```python
from build123d import *

# Parameters (mm, degrees)
F5_DEPTH = 25
F6_DEPTH = 25
F7_COUNT = 7


with BuildPart() as f5:
    # F3 (on Front) → F5 (new body)
    with BuildSketch(Plane.XZ):
        with BuildLine():
            ThreePointArc((-5, 29.5803989155), (-19.364916731, -22.9128784748), (30, 0))
            ThreePointArc((30, 0), (22.9128784748, 19.364916731), (5, 29.5803989155))
            ThreePointArc((5, 29.5803989155), (0, 30), (-5, 29.5803989155))
        make_face()
    extrude(amount=F5_DEPTH)



with BuildPart() as f6:
    # F3 (on Front) → F6 (new body)
    with BuildSketch(Plane.XZ):
        with BuildLine():
            ThreePointArc((-5, 29.5803989155), (0, 30), (5, 29.5803989155))
            Line((5, 29.5803989155), (1.0056277868, 30.2555710497))
            Line((1.0056277868, 30.2555710497), (0, 30.2555710497))
            Line((0, 30.2555710497), (-1.0056277868, 30.2555710497))
            Line((-1.0056277868, 30.2555710497), (-5, 29.5803989155))
        make_face()
    extrude(amount=F6_DEPTH)


with BuildPart() as f5_1:
    add(f5.part)

    add(f6.part)  # F7 merges F6
    # F7: F6, F5 ×7 about axis
    f7_axis = Axis((0, 33.5468817502, 0), (0, 1, 0))
    for i in range(1, F7_COUNT):
        add(f6.part.rotate(f7_axis, i * 360 / F7_COUNT))
        add(f5.part.rotate(f7_axis, i * 360 / F7_COUNT))


solid = f5_1.part
```
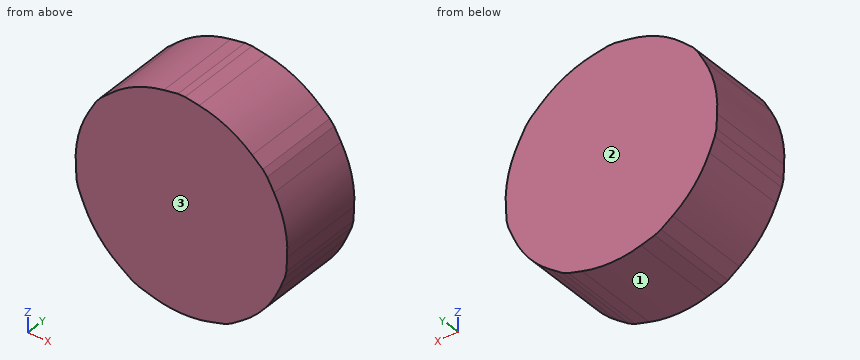
Design review of the part built by this model. Coordinates are the model's own, in mm. Face numbers are marked on the shaded views. Round coordinates to 2 decimals unless told otherwise and drop trailing zeros. Write each loop counter-clockwise with the first axis right and the second up, starting at its lowest first coordinate (ties: lowest second). Pieces come first, ordered by that corner, then holes.
Item 1: We need section B-B on x = 21. Write out the cut boundary in (y, z).
Item 2: Clearance check with flat-ended pins moving along their axes: pin 1 Ø10 at (y, z) = (-21, -15) entering from -X; pin 2 Ø6 at (x, y) = (21, -3) entering from +Z; pin 3 Ø10 at (y, z) = (-16, -10) entering from +X. State where each tip first meets the part, or that it passes through.
Item 3: For probe 1 along X at (y, z) = (-6.75, 14.5); probe 2 along X at (y, z) = (-14.5, 1.5); probe 3 along Z at (x, y) = (-3, -12.75), list the stretches that pass through material, from the lowest coordinate up.
Item 4: The part is to be moulded in two halves that separate along Y. For the marked faces 1, 2 and 3, say which applies: +Y half, -Y half, draft (parallel to the pull), parting line (faces both ways), or undercut.
Item 5: We need section C-C on z = -22. Write out the cut boundary in (x, y).
Item 6: We need section A-A on y = -22. Write out the cut boundary in (x, z).
Returned:
1. outline: (-25, -21.42) - (0, -21.42) - (0, 21.47) - (-25, 21.47) - close
2. pin 1: stops at x = -28.33
2. pin 2: stops at z = 24
2. pin 3: stops at x = 29.76
3. probe 1: x = -26.26 to 26.26
3. probe 2: x = -29.96 to 29.96
3. probe 3: z = -29.85 to 29.92
4. face 1: draft
4. face 2: +Y half
4. face 3: -Y half
5. outline: (-20.4, -25) - (20.4, -25) - (20.4, 0) - (-20.4, 0) - close
6. outline: (-29.95, -1.71) - (-29.72, -5.75) - (-29.27, -7.71) - (-27.73, -11.46) arc R30 ccw to (-17.34, -24.48) - (-14.03, -26.82) - (-12.22, -27.7) - (-8.33, -28.82) arc R30 ccw to (8.33, -28.82) - (12.22, -27.7) - (14.03, -26.82) - (17.34, -24.48) arc R30 ccw to (27.73, -11.46) - (29.27, -7.71) - (29.72, -5.75) - (29.95, -1.71) arc R30 ccw to (26.24, 14.53) - (24.28, 18.08) - (23.03, 19.65) - (20.01, 22.35) arc R30 ccw to (5, 29.58) - (1.01, 30.26) - (-1.01, 30.26) - (-5, 29.58) arc R30 ccw to (-20.01, 22.35) - (-23.03, 19.65) - (-24.28, 18.08) - (-26.24, 14.53) arc R30 ccw to start
